```python
from build123d import *

# Parameters (mm, degrees)
SKETCH1_R           = 3
BOSS_EXTRUDE1_DEPTH = 9.6
SKETCH2_R           = 1.75
CUT_EXTRUDE1_DEPTH  = 1
BOSS_EXTRUDE2_DEPTH = 3.75
SKETCH4_W           = 0.5
SKETCH4_H           = 1


with BuildPart() as part:
    # Sketch1 → Boss-Extrude1 (new body)
    with BuildSketch(Plane(origin=(0, 0, 0), x_dir=(1, 0, 0), z_dir=(0, 1, 0))):
        with Locations(Location((0, 0, 0), (0, 0, 270))):
            Circle(SKETCH1_R)
    extrude(amount=BOSS_EXTRUDE1_DEPTH)

    # Sketch2 → Cut-Extrude1 (cut)
    with BuildSketch(Plane.XZ):
        with Locations(Location((0, 0, 0), (0, 0, 270))):
            Circle(SKETCH2_R)
    extrude(amount=-CUT_EXTRUDE1_DEPTH, mode=Mode.SUBTRACT)

    # Sketch3 → Boss-Extrude2 (add)
    with BuildSketch(Plane(origin=(0, 9.6, 0), x_dir=(1, 0, 0), z_dir=(0, 1, 0))):
        with BuildLine():
            Line((-2.537715508, -1.6), (2.537715508, -1.6))
            ThreePointArc((2.537715508, -1.6), (3, 0), (2.537715508, 1.6))
            Line((2.537715508, 1.6), (-2.537715508, 1.6))
            ThreePointArc((-2.537715508, 1.6), (-3, 0), (-2.537715508, -1.6))
        make_face()
    extrude(amount=BOSS_EXTRUDE2_DEPTH)

    # Sketch4 → Cut-Revolve2 (revolve, cut)
    with BuildSketch(Plane(origin=(0, 0, 0), x_dir=(0, 0, -1), z_dir=(1, 0, 0)), mode=Mode.PRIVATE) as cut_revolve2_sk:
        with Locations((-2.75, 6.1)):
            Rectangle(SKETCH4_W, SKETCH4_H)
    revolve(cut_revolve2_sk.sketch.rotate(Axis((0, 0, 0), (0, 1, 0)), 180), axis=Axis((0, 0, 0), (0, 1, 0)), mode=Mode.SUBTRACT)


solid = part.part
```
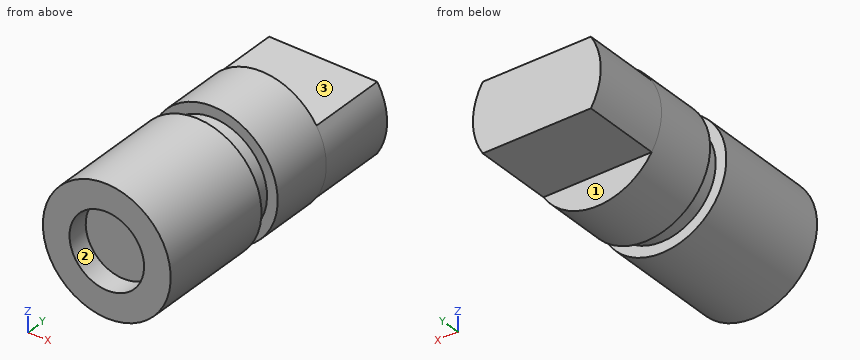
Input: part model. Units: mm. Frame: model coordinates. Face numbers are marked on the shaded views. A direction names the side the tool comes from. Round coordinates to 2 decimals unless told otherwise and drop trailing zeros. Loops run counter-clockwise (first coordinate to the right, second up) from the corner with the lowest first, then second, coordinate; pieces in that order, holes last. Notation, with made-up numbers: (13, 61) -> (30, 61) arc R13 cw to (30, 86) -> close; hole circle Ø7 at (39.25, 75). An arc over 180 degrees is marked (long way). Use one line per item in the form item = value. Start each with the question number.
Item 1: Section query A-A on z = 0. Return the cut outline in (x, y).
Item 2: Contact query for flat-ended pins moving along their axis: pin 1 Ø1.1 at (x, y) = (-0.5, 11.5) entering from -Z; pin 2 Ø1.8 at (x, z) = (0, -0.5) entering from -Y; pin 3 Ø0.7 at (x, z) = (1, 2.5) entering from +Y. Output: stop coordinate, or through.
Item 3: Section query C-C on y = 2.25. Return the cut outline in (x, z).
Item 4: Section query B-B on x = 0. Return the cut outline in (y, z).
Item 5: Material intervals for L1, parallel to X at y = 0.75, z = 0; L2, parallel to Y at x = -2.5, z = -1.2; L3, parallel to Y at x = -0.4, z = -2.65, sorted ascending. Write a range as from..to.
Item 6: Set-up query: the marked faces 1, 2 and 3. Return all of +Z, -Z, +X, -X, +Y, -Y with unobstructed straight access to the full face (end or side cutting, diameter ignored); none if empty.
Item 7: Section query D-D on z = 0.7. Return the cut outline in (x, y), then the cut area to 3 significant figures.
Ans:
q1.outline = (-3, 0) -> (-1.75, 0) -> (-1.75, 1) -> (1.75, 1) -> (1.75, 0) -> (3, 0) -> (3, 5.6) -> (2.5, 5.6) -> (2.5, 6.6) -> (3, 6.6) -> (3, 13.35) -> (-3, 13.35) -> (-3, 6.6) -> (-2.5, 6.6) -> (-2.5, 5.6) -> (-3, 5.6) -> close
q2.pin_1 = -1.6
q2.pin_2 = 1
q2.pin_3 = 9.6
q3.outline = circle Ø6 at (0, 0)
q4.outline = (0, -3) -> (5.6, -3) -> (5.6, -2.5) -> (6.6, -2.5) -> (6.6, -3) -> (9.6, -3) -> (9.6, -1.6) -> (13.35, -1.6) -> (13.35, 1.6) -> (9.6, 1.6) -> (9.6, 3) -> (6.6, 3) -> (6.6, 2.5) -> (5.6, 2.5) -> (5.6, 3) -> (0, 3) -> (0, 1.75) -> (1, 1.75) -> (1, -1.75) -> (0, -1.75) -> close
q5.L1 = -3..-1.75, 1.75..3
q5.L2 = 0..5.6, 6.6..13.35
q5.L3 = 0..5.6, 6.6..9.6
q6.face_1 = -Z, +X, -X, +Y
q6.face_2 = -Y
q6.face_3 = +Z, +X, -X, +Y
q7.outline = (-2.92, 0) -> (-1.6, 0) -> (-1.6, 1) -> (1.6, 1) -> (1.6, 0) -> (2.92, 0) -> (2.92, 5.6) -> (2.4, 5.6) -> (2.4, 6.6) -> (2.92, 6.6) -> (2.92, 13.35) -> (-2.92, 13.35) -> (-2.92, 6.6) -> (-2.4, 6.6) -> (-2.4, 5.6) -> (-2.92, 5.6) -> close
q7.area = 73.6 mm^2
